Autodesk Fusion 360 part; units mm, degrees
sketch "Sketch1" plane through (0, 0, 0) normal (0, 1, 0) x (1, 0, 0)
  line L0 (0, 0) -> (90, 0)
  line L1 (90, 0) -> (90, -40)
  line L2 (90, -40) -> (0, -40)
  line L3 (0, -40) -> (0, 0)
  dimension "d1" = 90
  dimension "d2" = 40
extrude "Extrude1" add sketch "Sketch1" along normal blind 30
sketch "Sketch2" plane through (0, 30, 0) normal (0, 1, 0) x (-1, 0, 0)
  line L0 (0, 40) -> (-90, 40)
  line L1 (-90, 40) -> (-90, 0)
  line L2 (-90, 0) -> (0, 0)
  line L3 (0, 0) -> (0, 40)
  line L4 (-85, 0) -> (-5, 0)
  line L5 (-5, 0) -> (-5, 35)
  line L6 (-5, 35) -> (-85, 35)
  line L7 (-85, 35) -> (-85, 0)
extrude "Extrude2" cut sketch "Sketch2" against normal blind 25 contours L2 L4 L5 L6 L7
sketch "Sketch3" plane through (0, 0, 0) normal (-1, 0, 0) x (0, -1, 0)
  line L0 (0, 0) -> (0, 40)
  line L1 (0, 40) -> (-30, 40)
  line L2 (-30, 40) -> (-30, 0)
  line L3 (-30, 0) -> (0, 0)
  line L4 (-25, 0) -> (-5, 0)
  line L5 (-5, 0) -> (-5, 10)
  line L6 (-5, 10) -> (-25, 10)
  line L7 (-25, 10) -> (-25, 0)
extrude "Extrude3" cut sketch "Sketch3" against normal blind 5 contours L3 L4 L5 L6 L7
sketch "Sketch4" plane through (0, 30, 0) normal (0, 1, 0) x (-1, 0, 0)
  line L0 (-85, 0) -> (-85, 35)
  line L1 (-85, 35) -> (-5, 35)
  line L2 (-5, 35) -> (-5, 0)
  line L3 (-5, 0) -> (0, 0)
  line L4 (0, 0) -> (0, 40)
  line L5 (0, 40) -> (-90, 40)
  line L6 (-90, 40) -> (-90, 0)
  line L7 (-90, 0) -> (-85, 0)
  line L8 (-90, 40) -> (-70, 40)
  line L9 (-70, 40) -> (-70, 35)
  line L10 (-70, 35) -> (-90, 35)
  line L11 (-90, 35) -> (-90, 40)
extrude "Extrude4" add sketch "Sketch4" along normal blind 30 contours L1 L5 L6 L8 L9 L10 L11
sketch "Sketch5" plane through (0, 0, 40) normal (0, 0, 1) x (-1, 0, 0)
  line L0 (0, 0) -> (-90, 0)
  line L1 (-90, 0) -> (-90, -60)
  line L2 (-90, -60) -> (-70, -60)
  line L3 (-70, -60) -> (-70, -30)
  line L4 (-70, -30) -> (0, -30)
  line L5 (0, -30) -> (0, 0)
  line L6 (-75.0796, -60) -> (-85.0796, -60)
  line L7 (-85.0796, -60) -> (-85.0796, -26)
  line L8 (-85.0796, -26) -> (-75.0796, -26)
  line L9 (-75.0796, -26) -> (-75.0796, -60)
  dimension "d11" = 10
  dimension "d12" = 34
extrude "Extrude5" cut sketch "Sketch5" against normal blind 5 contours L2 L6 L7 L8 L9
sketch "Sketch6" plane through (0, 5, 0) normal (0, 1, 0) x (-1, 0, 0)
  line L0 (-85, 35) -> (-85, 0)
  line L1 (-85, 0) -> (0, 0)
  line L2 (0, 0) -> (0, 10)
  line L3 (0, 10) -> (-5, 10)
  line L4 (-5, 10) -> (-5, 35)
  line L5 (-5, 35) -> (-85, 35)
  line L6 (-80, 25) -> (-71, 25)
  line L7 (-71, 16) -> (-71, 0)
  line L8 (-71, 0) -> (-80, 0)
  line L9 (-80, 0) -> (-80, 25)
  line L10 (-80, 25) -> (-63, 25)
  line L11 (-63, 16) -> (-71, 16)
  line L12 (-80, 16) -> (-80, 25)
  line L13 (-50, 28) -> (-33, 28)
  line L14 (-33, 28) -> (-33, 18)
  line L15 (-33, 18) -> (-50, 18)
  line L16 (-50, 18) -> (-50, 28)
  arc A0 (-63, 16) -> (-63, 25) centre (-63, 20.5) ccw
  dimension "d15" = 9
  dimension "d16" = 17
extrude "Extrude6" cut sketch "Sketch6" against normal blind 5 contours L1 L6 L7 L8 L9 L10 L11 L12 A0
sketch "Sketch7" plane through (0, 5, 0) normal (0, 1, 0) x (-1, 0, 0)
  line L0 (-80, 0) -> (-80, 25)
  line L1 (-80, 25) -> (-63, 25)
  arc A0 (-63, 16) -> (-63, 25) centre (-63, 20.5) ccw
  line L2 (-63, 16) -> (-71, 16)
  line L3 (-71, 16) -> (-71, 0)
  line L4 (-71, 0) -> (0, 0)
  line L5 (0, 0) -> (0, 10)
  line L6 (0, 10) -> (-5, 10)
  line L7 (-5, 10) -> (-5, 35)
  line L8 (-5, 35) -> (-85, 35)
  line L9 (-85, 35) -> (-85, 0)
  line L10 (-85, 0) -> (-80, 0)
  line L11 (-12, 28) -> (-29, 28)
  line L12 (-29, 28) -> (-29, 18)
  line L13 (-29, 18) -> (-12, 18)
  line L14 (-12, 18) -> (-12, 28)
extrude "Extrude7" cut sketch "Sketch7" against normal blind 8 contours L11 L12 L13 L14
sketch "Sketch8" plane through (0, 5, 0) normal (0, 1, 0) x (-1, 0, 0)
  line L0 (-29, 28) -> (-12, 28)
  line L1 (-12, 28) -> (-12, 18)
  line L2 (-12, 18) -> (-29, 18)
  line L3 (-29, 18) -> (-29, 28)
  line L4 (-80, 0) -> (-80, 25)
  line L5 (-80, 25) -> (-63, 25)
  arc A0 (-63, 16) -> (-63, 25) centre (-63, 20.5) ccw
  line L6 (-63, 16) -> (-71, 16)
  line L7 (-71, 16) -> (-71, 0)
  line L8 (-71, 0) -> (0, 0)
  line L9 (0, 0) -> (0, 10)
  line L10 (0, 10) -> (-5, 10)
  line L11 (-5, 10) -> (-5, 35)
  line L12 (-5, 35) -> (-85, 35)
  line L13 (-85, 35) -> (-85, 0)
  line L14 (-85, 0) -> (-80, 0)
  line L15 (-35, 28) -> (-52, 28)
  line L16 (-52, 28) -> (-52, 18)
  line L17 (-52, 18) -> (-35, 18)
  line L18 (-35, 18) -> (-35, 28)
extrude "Extrude8" cut sketch "Sketch8" against normal blind 6 contours L15 L16 L17 L18
sketch "Sketch9" plane through (0, 5, 0) normal (0, 1, 0) x (-1, 0, 0)
  line L0 (-52, 28) -> (-35, 28)
  line L1 (-35, 28) -> (-35, 18)
  line L2 (-35, 18) -> (-52, 18)
  line L3 (-52, 18) -> (-52, 28)
  line L4 (-29, 28) -> (-12, 28)
  line L5 (-12, 28) -> (-12, 18)
  line L6 (-12, 18) -> (-29, 18)
  line L7 (-29, 18) -> (-29, 28)
  line L8 (-80, 0) -> (-80, 25)
  line L9 (-80, 25) -> (-63, 25)
  arc A0 (-63, 16) -> (-63, 25) centre (-63, 20.5) ccw
  line L10 (-63, 16) -> (-71, 16)
  line L11 (-71, 16) -> (-71, 0)
  line L12 (-71, 0) -> (0, 0)
  line L13 (0, 0) -> (0, 10)
  line L14 (0, 10) -> (-5, 10)
  line L15 (-5, 10) -> (-5, 35)
  line L16 (-5, 35) -> (-85, 35)
  line L17 (-85, 35) -> (-85, 0)
  line L18 (-85, 0) -> (-80, 0)
  line L19 (-54, 30) -> (-33, 30)
  line L20 (-33, 30) -> (-33, 15)
  line L21 (-33, 15) -> (-54, 15)
  line L22 (-54, 15) -> (-54, 30)
extrude "Extrude9" add sketch "Sketch9" along normal blind 20 contours L19 L20 L21 L22
sketch "Sketch10" plane through (0, 5, 0) normal (0, 1, 0) x (-1, 0, 0)
  line L0 (-54, 15) -> (-54, 30)
  line L1 (-54, 30) -> (-33, 30)
  line L2 (-33, 30) -> (-33, 15)
  line L3 (-33, 15) -> (-54, 15)
  line L4 (-29, 28) -> (-12, 28)
  line L5 (-12, 28) -> (-12, 18)
  line L6 (-12, 18) -> (-29, 18)
  line L7 (-29, 18) -> (-29, 28)
  line L8 (-80, 0) -> (-80, 25)
  line L9 (-80, 25) -> (-63, 25)
  arc A0 (-63, 16) -> (-63, 25) centre (-63, 20.5) ccw
  line L10 (-63, 16) -> (-71, 16)
  line L11 (-71, 16) -> (-71, 0)
  line L12 (-71, 0) -> (0, 0)
  line L13 (0, 0) -> (0, 10)
  line L14 (0, 10) -> (-5, 10)
  line L15 (-5, 10) -> (-5, 35)
  line L16 (-5, 35) -> (-85, 35)
  line L17 (-85, 35) -> (-85, 0)
  line L18 (-85, 0) -> (-80, 0)
  line L19 (-31, 30) -> (-10, 30)
  line L20 (-10, 30) -> (-10, 15)
  line L21 (-10, 15) -> (-31, 15)
  line L22 (-31, 15) -> (-31, 30)
extrude "Extrude10" add sketch "Sketch10" along normal blind 20 contours L19 L20 L21 L22
sketch "Sketch11" plane through (0, 0, 0) normal (-1, 0, 0) x (0, -1, 0)
  line L0 (-25, 0) -> (-25, 10)
  line L1 (-25, 10) -> (-5, 10)
  line L2 (-5, 10) -> (-5, 0)
  line L3 (-5, 0) -> (0, 0)
  line L4 (0, 0) -> (0, 40)
  line L5 (0, 40) -> (-30, 40)
  line L6 (-30, 40) -> (-30, 0)
  line L7 (-30, 0) -> (-25, 0)
  line L8 (-25, 0) -> (-30, 0)
  line L9 (-30, 0) -> (-30, 18)
  line L10 (-30, 18) -> (-25, 18)
  line L11 (-25, 18) -> (-25, 0)
  dimension "d27" = 18
extrude "Extrude11" add sketch "Sketch11" against normal blind 54 contours L0 L6 L7 L8 L9 L10 L11
sketch "Sketch12" plane through (0, 0, 15) normal (0, 0, -1) x (1, 0, 0)
  line L0 (54, -5) -> (33, -5)
  line L1 (33, -5) -> (33, -25)
  line L2 (33, -25) -> (54, -25)
  line L3 (54, -25) -> (54, -5)
  circle A0 centre (43.5, -17.5) radius 1.5
  circle A1 centre (20, -17.5) radius 1.5
  line L4 (54, -25) -> (0, -25)
  dimension "d30" = 7.5
  dimension "d31" = 3
  dimension "d32" = 7.5
  dimension "d33" = 3
extrude "Extrude12" cut sketch "Sketch12" against normal blind 4 contours A0
sketch "Sketch13" plane through (0, 0, 15) normal (0, 0, -1) x (1, 0, 0)
  line L0 (31, -5) -> (10, -5)
  line L1 (10, -5) -> (10, -25)
  line L2 (10, -25) -> (31, -25)
  line L3 (31, -25) -> (31, -5)
  circle A0 centre (20, -17.5) radius 1.5
  dimension "d36" = 7.5
  dimension "d37" = 3
  dimension "d38" = 11
extrude "Extrude13" cut sketch "Sketch13" against normal blind 4 contours A0
sketch "Sketch14" plane through (0, 30, 0) normal (0, 1, 0) x (-1, 0, 0)
  line L0 (0, 0) -> (0, 40)
  line L1 (0, 40) -> (-70, 40)
  line L2 (-70, 40) -> (-70, 35)
  line L3 (-70, 35) -> (-5, 35)
  line L4 (-5, 35) -> (-5, 18)
  line L5 (-5, 18) -> (-54, 18)
  line L6 (-54, 18) -> (-54, 0)
  line L7 (-54, 0) -> (0, 0)
  line L8 (-54, 10) -> (-31, 10)
  line L9 (-31, 10) -> (-31, 0)
  line L10 (-31, 0) -> (-54, 0)
  line L11 (-54, 0) -> (-54, 10)
  dimension "d41" = 10
extrude "Extrude14" cut sketch "Sketch14" against normal blind 5 contours L6 L7 L8 L9 L10 L11
sketch "Sketch15" plane through (0, 0, 35) normal (0, 0, -1) x (1, 0, 0)
  line L0 (75.0796, -26) -> (85, -26)
  line L1 (85, -26) -> (85, -5)
  line L2 (85, -5) -> (5, -5)
  line L3 (5, -5) -> (5, -30)
  line L4 (5, -30) -> (70, -30)
  line L5 (70, -30) -> (70, -60)
  line L6 (70, -60) -> (75.0796, -60)
  line L7 (75.0796, -60) -> (75.0796, -26)
  line L8 (75.0796, -26) -> (70, -26)
  line L9 (70, -26) -> (70, -60)
  line L10 (70, -60) -> (75.0796, -60)
  line L11 (75.0796, -60) -> (75.0796, -26)
extrude "Extrude15" add sketch "Sketch15" along normal blind 5 contours L5 L6 L7 L8 L9 L10 L11
extrude "Extrude16" add 1 faces at (88.3599, 50, 35) along direction (0, 0, -1) blind 5
sketch "Sketch16" plane through (0, 60, 0) normal (0, 1, 0) x (-1, 0, 0)
  line L0 (-85.0796, 30) -> (-85.0796, 40)
  line L1 (-85.0796, 40) -> (-90, 40)
  line L2 (-90, 40) -> (-90, 30)
  line L3 (-90, 30) -> (-85.0796, 30)
sketch "Sketch17" plane through (0, 0, 30) normal (0, 0, -1) x (1, 0, 0)
  line L0 (75.0796, -60) -> (75.0796, -26)
  line L1 (75.0796, -26) -> (70, -26)
  line L2 (70, -26) -> (70, -60)
  line L3 (70, -60) -> (75.0796, -60)
  line L4 (75.0796, -26) -> (70, -26)
  line L5 (70, -26) -> (70, -21)
  line L6 (70, -21) -> (75.0796, -21)
  line L7 (75.0796, -21) -> (75.0796, -26)
extrude "Extrude17" add sketch "Sketch17" against normal blind 5 contours L1 L4 L5 L6 L7
fillet "Fillet1" radius 2 1 edges at (90, 0, 20)
fillet "Fillet2" radius 2 3 edges at (90, 31, 40) (89.4142, 0.5858, 40) (44, 0, 40)
fillet "Fillet3" radius 2 3 edges at (0, 16, 40) (0, 0.5858, 39.4142) (0, 0, 19)
fillet "Fillet4" radius 2 3 edges at (0, 30, 19) (0.5858, 30, 39.4142) (36, 30, 40)
fillet "Fillet5" radius 2 1 edges at (70, 44, 40)
fillet "Fillet6" radius 2 1 edges at (80, 2.5, 25)
fillet "Fillet7" radius 2 1 edges at (71, 2.5, 16)
Verification items for the finished model (mm, model axes). A direction names the side the tool comes from. Round coordinates to 2 decimals unless told otherwise and drop trailing zeros. Loops run counter-clockwise (first coordinate to the right, second up) from the corner with the lowest first, then second, coordinate; pieces in that order, holes last. Notation, with made-up numbers: (-23, 48) -> (29, 48) arc R14 cw to (29, 67) -> close; hole circle Ø8 at (-27, 51.25). An arc over 180 degrees is marked (long way). Answer as a JSON object with one key per item and string values.
Q1. Section check B-B (x = 43.5). Record the boundary of the cut face in (y, z).
Data:
{"outline": "(0, 0) -> (5, 0) -> (5, 15) -> (16, 15) -> (16, 18) -> (0, 18) -> close; (0, 28) -> (25, 28) -> (25, 30) -> (5, 30) -> (5, 35) -> (30, 35) -> (30, 38) arc R2 ccw to (28, 40) -> (2, 40) arc R2 ccw to (0, 38) -> close; (19, 15) -> (25, 15) -> (25, 10) -> (30, 10) -> (30, 18) -> (19, 18) -> close"}
Q2. Go/stop test with flat-tipped pins: P1, Ø6, axis at x = 67.5, y = 35, coming from the -Z side; P2, Ø9.5, axis at x = 22, z = 24.5, coming from the +Y side; P3, Ø6, axis at x = 21, y = 12.5, coming from the -Z side. Record where each tip stops, or that it passes through.
Data:
{"P1": "stops at z = 30", "P2": "stops at y = 25", "P3": "stops at z = 15"}
Q3. Scan lines: line 1 (Y direction, x = 43.5, z = 16.15); line 2 (Z direction, x = 25, y = 3.5); line 3 (Y direction, x = 18.5, z = 9). Record each from-to range of solid material in increasing order. Write a range as from..to.
Data:
{"line 1": "y = 0..16, 19..30", "line 2": "z = 0..18, 28..40", "line 3": "y = 0..5, 25..30"}
Q4. Access from +Z, -Z, +X, -X, +Y, -Y to the whole of each face (thin tool, end or side, straight path). Record for faces 1 (the flat face through (28, 30, 15)), 2 (the cylindrical face through (18.89, 16.49, 16.48)), 3 (the flat face through (35, 12, 23)).
Data:
{"face 1": "+Z, -Z, -X, +Y", "face 2": "-Z", "face 3": "+Y, -Y"}
Q5. Draft check along Y on faces 4 (the flat face through (44, 0, 15)), 5 (the flat face through (44, 25, 29)), 6 (the flat face through (5, 18, 22)). Enter one of: pulls with the +Y half, pulls with the -Y half, needs draft (parallel to the pull), parting line crosses it, or undercut.
Data:
{"face 4": "pulls with the -Y half", "face 5": "pulls with the +Y half", "face 6": "undercut"}
Q6. Section check A-A (z = 20.5). State how many separate pieces and enclosed holes the cut face has, then the cut area to 3 significant figures.
Data:
{"separate pieces": "4", "enclosed holes": "0", "area": "580 mm2"}
Q7. Section check D-D (x = 17). Record the boundary of the cut face in (y, z).
Data:
{"outline": "(0, 0) -> (5, 0) -> (5, 15) -> (25, 15) -> (25, 0) -> (30, 0) -> (30, 18) -> (0, 18) -> close; (0, 28) -> (25, 28) -> (25, 30) -> (5, 30) -> (5, 35) -> (30, 35) -> (30, 38) arc R2 ccw to (28, 40) -> (2, 40) arc R2 ccw to (0, 38) -> close"}
